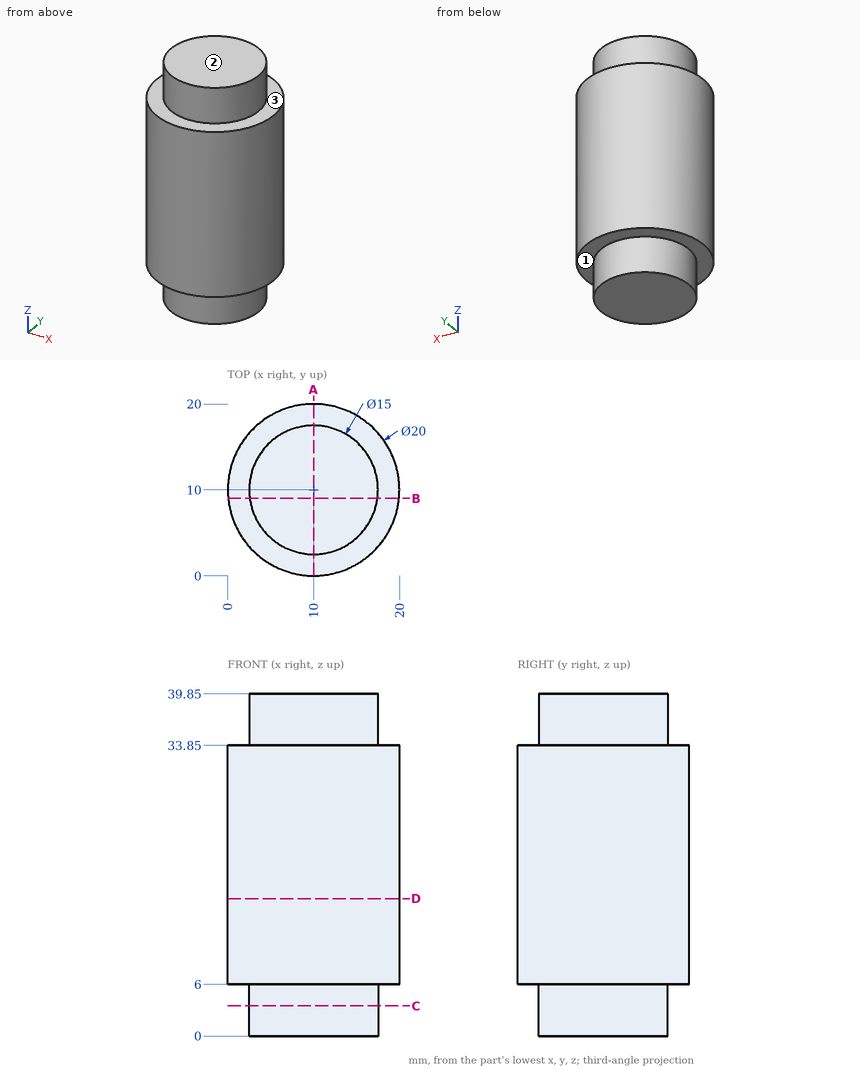
Study the drawing (mm; zero at the part's minimum x, y, z) and answer. A direction names the side the tool comes from. Give positions to 0.01 mm unless a question says otherwise; leave off trailing zeros. Write each loop counter-clockwise with the first axis right and the second up, starting at its lowest first coordinate (ties: lowest second). Pieces come first, ordered by that corner, then holes. Notation, with made-up numbers: M 7,26 L 26,26 A13 cw 26,40 Z; hole C -12.5,-22 d3. An arc over 180 degrees is marked long. Put each result on its own line as item: value. Start each with the question number.
1. Consider line 1 along Z through (x, y) = (12.75, 17.25); line 2 along X through (y, z) = (9.75, 3); line 3 along X through (y, z) = (13.25, 19.5). Determine where each line is inside the solid, lowest interval first.
2. The part is cut by section D-D, the plane z = 16. Give the vertices of the cut face in (x, y).
3. The part is cut by section A-A, the plane x = 10. Give the vertices of the cut face in (y, z), and give its area (3 significant figures).
4. The part is cut by section B-B, the plane y = 9. Give the vertices of the cut face in (x, z), and give its area (3 significant figures).
5. The part is cut by section C-C, the plane z = 3.5. Give the vertices of the cut face in (x, y), and give its area (3 significant figures).
6. Which of the six approach directions +Z, -Z, +X, -X, +Y, -Y give full straight-line access (tool end or side, diameter ignored) to the marked faces 1, 2 and 3?
7. Each of these flat-tipped pins is pushed along its axis until it touches: pin 1 Ø4 at (y, z) = (5, 15.5) entering from -X; pin 2 Ø2 at (x, z) = (3, 10) entering from -Y; pin 3 Ø12 at (y, z) = (17, 21) entering from -X. Where does it stop, or does it pass through?
Final values:
1. line 1: z = 6 to 33.85
1. line 2: x = 2.5 to 17.5
1. line 3: x = 0.54 to 19.46
2. outline: C 10,10 d20
3. outline: M 0,6 L 2.5,6 L 2.5,0 L 17.5,0 L 17.5,6 L 20,6 L 20,33.85 L 17.5,33.85 L 17.5,39.85 L 2.5,39.85 L 2.5,33.85 L 0,33.85 Z
3. area: 737 mm²
4. outline: M 0.05,6 L 2.57,6 L 2.57,0 L 17.43,0 L 17.43,6 L 19.95,6 L 19.95,33.85 L 17.43,33.85 L 17.43,39.85 L 2.57,39.85 L 2.57,33.85 L 0.05,33.85 Z
4. area: 733 mm²
5. outline: C 10,10 d15
5. area: 177 mm²
6. face 1: -Z
6. face 2: +Z, +X, -X, +Y, -Y
6. face 3: +Z
7. pin 1: stops at x = 0.46
7. pin 2: stops at y = 2
7. pin 3: stops at x = 0.05
